Source: three-view drawing plus pictorial views. Frame: mm from the lowest corner of the part. A direction names the side the tool comes from. Give positions to 0.01 mm unless a question says otherwise; leave off trailing zeros. Order: outer loops, then holes, each group sorted by start corner. A loop starts at its lowest first (then second) coordinate and runs counter-clockwise, first axis right, second up. Notation, with made-up numbers: (5.5, 63.25) -> (62.5, 63.25) arc R27 ccw to (62.5, 100.25) -> close; hole circle Ø1 at (2.25, -11). An arc over 180 degrees is marked (long way). Answer in a Markdown table with one row per item. Add a question column.
Q1. Line query: line 1 along X through (y, z) = (17, 15.5); line 2 along Z through (x, y) = (10.5, 7). Output: solid intervals per line, ascending. Write a range as from..to.
Q2. Cut plane C-C on x = 22.5. Return the cut outline in (y, z).
Q3. Cut plane D-D on z = 14. Return the cut outline in (x, y), and give its area (3 significant figures).
Q4. Contact query for flat-ended pins moving along their axis: P1, Ø4, axis at y = 25, z = 29.5, coming from the -X side; P2, Ø12, axis at x = 20.5, z = 20, coming from the -Y side; P3, Ø5, axis at x = 7.07, y = 7.07, coming from the +Z side; P4, Ø9, axis at x = 22.5, y = 9.5, coming from the +Z side. Output: stop coordinate, or through.
Q5. Cut plane A-A on x = 8. Return the cut outline in (y, z), and give its area (3 significant figures).
Q6. Set-up query: the marked faces 1 and 2. Return all of +Z, -Z, +X, -X, +Y, -Y with unobstructed straight access to the full face (end or side cutting, diameter ignored); none if empty.
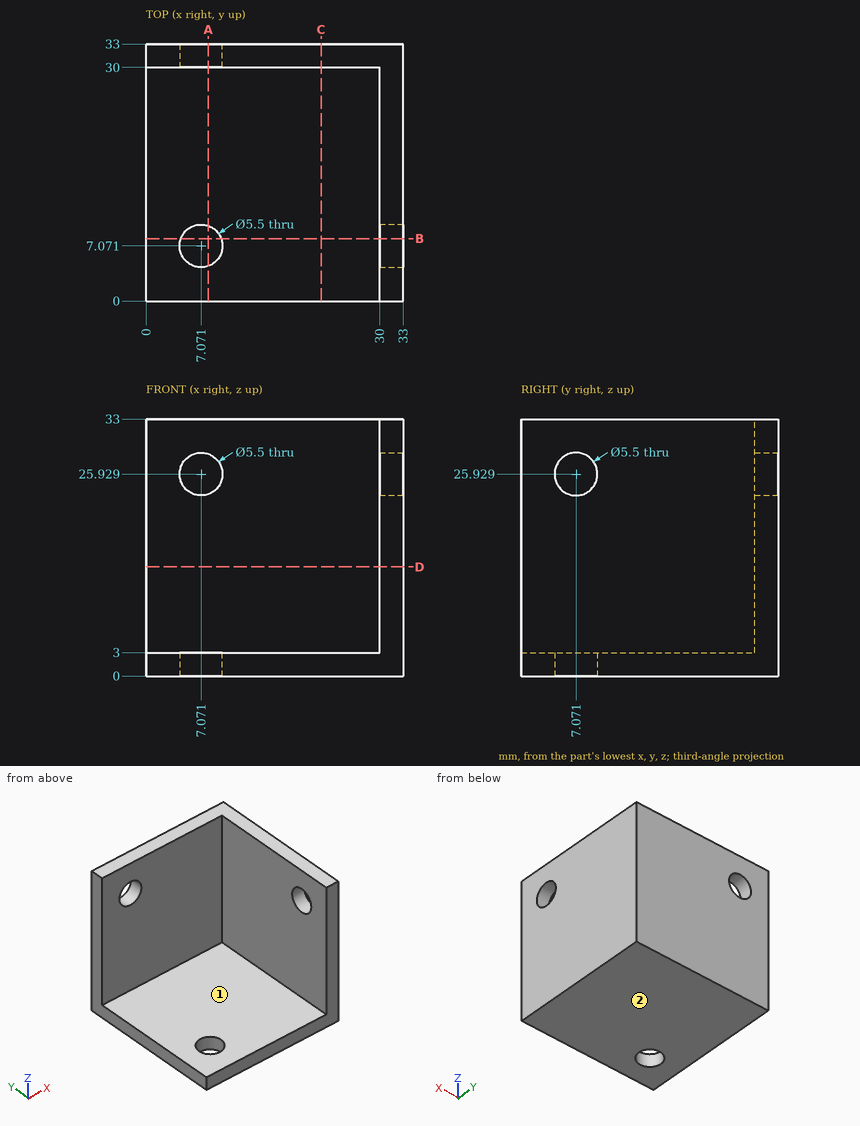
Completed:
| question | item | result |
|---|---|---|
| 1 | line 1 | x = 30..33 |
| 1 | line 2 | z = 0..3 |
| 2 | outline | (0, 0) -> (33, 0) -> (33, 33) -> (30, 33) -> (30, 3) -> (0, 3) -> close |
| 3 | outline | (0, 30) -> (30, 30) -> (30, 0) -> (33, 0) -> (33, 33) -> (0, 33) -> close |
| 3 | area | 189 mm² |
| 4 | P1 | stops at x = 30 |
| 4 | P2 | stops at y = 30 |
| 4 | P3 | passes through |
| 4 | P4 | stops at z = 3 |
| 5 | outline | (0, 0) -> (4.48, 0) -> (4.48, 3) -> (0, 3) -> close; (9.66, 0) -> (33, 0) -> (33, 23.34) -> (30, 23.34) -> (30, 3) -> (9.66, 3) -> close; (30, 28.52) -> (33, 28.52) -> (33, 33) -> (30, 33) -> close |
| 5 | area | 158 mm² |
| 6 | face 1 | +Z, -X, -Y |
| 6 | face 2 | -Z, +X, -X, +Y, -Y |
